Model file for the job. Use its own axes, mm. A direction names the side the tool comes from. Round coordinates to 2 decimals unless told otherwise and drop trailing zeros. Loops run counter-clockwise (first coordinate to the right, second up) from the corner with the lowest first, then second, coordinate; pieces in that order, holes last. Notation, with made-up numbers: M 37.5,30 L 63.5,30 A15 cw 63.5,52 Z; hole C 45.5,-23 d4. An arc over 180 degrees is marked long. Use a Markdown table: item, result. Add a question column.
Q1. Pin check, flat tips, straight feed: pin 1 (2 mm diameter, centred on x = -49, y = 0, fed in from +Z); pin 2 (1.5 mm diameter, centred on x = 0, y = 0, fed in from -Z); pin 3 (7 mm diameter, centred on x = -30, z = 25, fed in from +Y). Stop position of each tip, or through.
Q2. Probe line 1 (X direction, y = 0, z = 5.5); line 2 (Z direction, x = -30, y = -2.8); line 3 (Y direction, x = 49, z = 34). List the from-to ranges inside material, lowest first. Write a range as from..to.
Q3. Cut at C-C (z = 5.5). Give the cut face in (x, y), plus the area to 3 significant figures.
Q4. Tool access for faces 1 (the face through (-37.5, 1, 25)), 2 (the face through (6.8, 0, 24.9)), 3 (the face through (48.81, -0.1, 28.39)), 4 (the face through (-1, 4, 18)), 5 (the face through (0.748, -0.976, 4.056)): list every direction of +Z, -Z, +X, -X, +Y, -Y with a clear straight run to the whole face (end or side of a thin tool).
Q5. Cut at A-A (x = -30). Give the cut face in (y, z), plus the area to 3 significant figures.
Q6. Mould opens along Y. For faces 6 (the face through (-49.21, 0.05, 28.39)), 7 (the face through (46.17, 3.64, 18.85)), 8 (the face through (-30, 1, 32.5)) say: +Y half, -Y half, draft (parallel to the pull), parting line (faces both ways), or undercut.
Q7. Cut at B-B (z = 25). Give the cut face in (x, y).
Autodesk Inventor part; units mm, degrees
ref_plane "YZ Plane" through (0, 0, 0) normal (1, 0, 0) x (0, 1, 0)
ref_plane "XZ Plane" through (0, 0, 0) normal (0, 1, 0) x (-1, 0, 0)
ref_plane "XY Plane" through (0, 0, 0) normal (0, 0, 1) x (1, 0, 0)
sketch "Sketch1" plane through (0, 0, 0) normal (0, 0, 1) x (1, 0, 0)
  line L0 (-55, 4) -> (55, 4)
  line L1 (55, 4) -> (55, -4)
  line L2 (55, -4) -> (-55, -4)
  line L3 (-55, -4) -> (-55, 4)
  line L4 (-55, 4) -> (55, -4) construction
  line L5 (55, 4) -> (-55, -4) construction
  point P0 (0, 0)
  dimension "d0" = 110
  dimension "d1" = 8
extrude "Extrusion1" add sketch "Sketch1" along normal blind 37
sketch "Sketch2" plane through (0, 0, 37) normal (0, 0, 1) x (1, 0, 0)
  line L0 (-55, 4) -> (-55, -4)
  line L1 (55, -4) -> (55, 4)
  point P0 (0, 0)
  point P1 (-49, 0)
  point P2 (0, 0)
  point P3 (49, 0)
  dimension "d4" = 6
  dimension "d5" = 6
hole "Hole1" at (-49, 0, 37) at (0, 0, 37) at (49, 0, 37) direction (0, 0, -1) diameter 2.459 depth 8 tip angle 118
fillet "Fillet1" [suppressed]
sketch "Sketch3" plane through (0, 0, 0) normal (0, 0, -1) x (-1, 0, 0)
  circle A0 centre (-49, 0) radius 1.2295
  circle A1 centre (0, 0) radius 1.2295
  circle A2 centre (49, 0) radius 1.2295
hole "Hole2" at (49, 0, 0) at (0, 0, 0) at (-49, 0, 0) direction (0, 0, 1) diameter 2.459 depth 8 tip angle 118
sketch "Sketch6" plane through (-55, -4, 0) normal (0, -1, 0) x (1, 0, 0)
  line L0 (89.5, 18.5) -> (101.5, 18.5)
  line L1 (101.5, 18.5) -> (101.5, 31)
  line L2 (101.5, 31) -> (89.5, 31)
  line L3 (89.5, 31) -> (89.5, 18.5)
  line L4 (110, 0) -> (110, 37)
  line L5 (110, 0) -> (0, 0)
  line L6 (0, 37) -> (110, 37)
  point P0 (55, 0)
  dimension "d34" = 8.5
  dimension "d35" = 12
  dimension "d61" = 6
  dimension "d62" = 12.5
extrude "Extrusion3" cut sketch "Sketch6" against normal blind 10
fillet "Fillet2" radius 1.5 4 edges at (34.5, 0, 31) (46.5, 0, 31) (46.5, 0, 18.5) (34.5, 0, 18.5)
sketch "Sketch7" plane through (-55, 4, 0) normal (0, 1, 0) x (1, 0, 0)
  circle A0 centre (25, -25) radius 4
  line L0 (110, -37) -> (0, -37)
  line L1 (110, 0) -> (110, -37)
  point P0 (55, 0)
  dimension "d44" = 8
  dimension "d45" = 12
  dimension "d46" = 85
extrude "Extrusion4" cut sketch "Sketch7" against normal blind 10
sketch "Sketch9" plane through (-55, 4, 0) normal (0, 1, 0) x (1, 0, 0)
  line L0 (32.5, -32.5) -> (17.5, -32.5)
  line L1 (17.5, -32.5) -> (17.5, -17.5)
  line L2 (17.5, -17.5) -> (32.5, -17.5)
  line L3 (32.5, -17.5) -> (32.5, -32.5)
  circle A0 centre (25, -25) radius 4
  line L4 (32.5, -32.5) -> (17.5, -17.5) construction
  line L5 (17.5, -32.5) -> (32.5, -17.5) construction
  point P0 (55, 0)
  dimension "d52" = 15
  dimension "d53" = 15
extrude "Extrusion6" cut sketch "Sketch9" against normal blind 6
fillet "Fillet3" radius 2 4 edges at (-22.5, 1, 32.5) (-22.5, 1, 17.5) (-37.5, 1, 17.5) (-37.5, 1, 32.5)
chamfer "Chamfer3" distance 0.5 angle 45 16 edges at (40.5, 4, 31) (34.9393, 4, 30.5607) (34.5, 4, 24.75) (34.9393, 4, 18.9393) (40.5, 4, 18.5) (46.0607, 4, 18.9393) (46.5, 4, 24.75) (46.0607, 4, 30.5607) (-30, 4, 17.5) (-23.0858, 4, 18.0858) (-22.5, 4, 25) (-23.0858, 4, 31.9142) (-30, 4, 32.5) (-36.9142, 4, 31.9142) (-37.5, 4, 25) (-36.9142, 4, 18.0858)
sketch "Sketch10" plane through (-55, 4, 0) normal (0, 1, 0) x (1, 0, 0)
  line L0 (110, 0) -> (110, -37)
  line L1 (70.5, -30.6736) -> (65.5, -30.6736)
  line L2 (65.5, -19.3264) -> (70.5, -19.3264)
  line L3 (70.5, -30.6736) -> (65.5, -19.3264) construction
  line L4 (65.5, -30.6736) -> (70.5, -19.3264) construction
  arc A0 (70.5, -30.6736) -> (70.5, -19.3264) centre (68, -25) ccw
  arc A1 (65.5, -19.3264) -> (65.5, -30.6736) centre (68, -25) ccw
  point P0 (55, 0)
  dimension "d70" = 42
  dimension "d74" = 5
extrude "Extrusion7" cut sketch "Sketch10" against normal blind 10
chamfer "Chamfer4" [suppressed]
fillet "Fillet5" radius 1.5 4 edges at (15.5, 0, 30.6736) (10.5, 0, 30.6736) (15.5, 0, 19.3264) (10.5, 0, 19.3264)
chamfer "Chamfer5" distance 0.5 angle 45 16 edges at (13, 4, 19.3264) (15.5162, 4, 19.369) (19.2, 4, 25) (15.5162, 4, 30.631) (13, 4, 30.6736) (10.4838, 4, 30.631) (6.8, 4, 25) (10.4838, 4, 19.369) (19.2, -4, 25) (15.5162, -4, 19.369) (13, -4, 19.3264) (10.4838, -4, 19.369) (6.8, -4, 25) (10.4838, -4, 30.631) (13, -4, 30.6736) (15.5162, -4, 30.631)
properties part number "back accses panel" material "Aluminum 6061"
Checked values:
| question | item | result |
|---|---|---|
| 1 | pin 1 | stops at z = 28.86 |
| 1 | pin 2 | stops at z = 8.29 |
| 1 | pin 3 | passes through |
| 2 | line 1 | x = -55..-50.23, -47.77..-1.23, 1.23..47.77, 50.23..55 |
| 2 | line 2 | z = 0..21, 29..37 |
| 2 | line 3 | y = -4..-1.23, 1.23..4 |
| 3 | outline | M -55,-4 L 55,-4 L 55,4 L -55,4 Z; hole C -49,0 d2.46; hole C 0,0 d2.46; hole C 49,0 d2.46 |
| 3 | area | 866 mm^2 |
| 4 | face 1 | +Y |
| 4 | face 2 | +Y, -Y |
| 4 | face 3 | +Z |
| 4 | face 4 | +Z, -Z, +X, -X, +Y |
| 4 | face 5 | -Z |
| 5 | outline | M -4,0 L 4,0 L 4,17 L 3.5,17.5 L -2,17.5 L -2,21 L -4,21 Z; M -4,29 L -2,29 L -2,32.5 L 3.5,32.5 L 4,33 L 4,37 L -4,37 Z |
| 5 | area | 190 mm^2 |
| 6 | face 6 | undercut |
| 6 | face 7 | +Y half |
| 6 | face 8 | draft |
| 7 | outline | M -55,-4 L -34,-4 L -34,-2 L -37.5,-2 L -37.5,3.5 L -38,4 L -55,4 Z; M -26,-4 L 6.3,-4 L 6.8,-3.5 L 6.8,3.5 L 6.3,4 L -22,4 L -22.5,3.5 L -22.5,-2 L -26,-2 Z; M 19.2,-3.5 L 19.7,-4 L 34.5,-4 L 34.5,3.5 L 34,4 L 19.7,4 L 19.2,3.5 Z; M 46.5,-4 L 55,-4 L 55,4 L 47,4 L 46.5,3.5 Z |
